Could you check a few things on this drawing? It's one solid part, dimensions in mm from its lowest x, y, z. Give positions to 0.01 mm unless a question says otherwise; leave off trailing zeros. Order: outer loops, then holes, each group sorted by start corner. A loop starts at its lowest first (then second) coordinate and runs counter-clockwise, first axis right, second up. Notation, with made-up numbers: (15.25, -37) -> (70.25, -37) arc R31 ccw to (70.25, -6) -> close; hole circle Ø10 at (61, 6). An arc over 180 degrees is marked (long way). Write each question's results on one line, items separated by ' | '. Start each with the question number.
Q1. I'm going to push flat-ended pins straight in: pin 1 (2 mm diameter, centred on x = 16, y = 23, fed in from +Z); pin 2 (1.5 mm diameter, centred on x = 64.5, y = 63.5, fed in from +Z). Where does each tip first touch, or does it pass through?
Q2. Imagine slicing it at C-C, the plane z = 0.8. Please give me the cut outline in (x, y).
Q3. Thinking about a two-plate mould opening in X: for the marked faces 1 and 2, which applies, pulls with the +X half, pulls with the -X half, needs draft (parallel to the pull), parting line crosses it, or undercut?
Q4. I need wall thicknesses on line 1 along X through (y, z) = (39, 0.65); line 2 along Y through (x, z) = (40, 0.95); line 3 along X through (y, z) = (15.5, 3.7). Which ranges of each line are inside material? Lowest first, please. Write a range as [from, to].
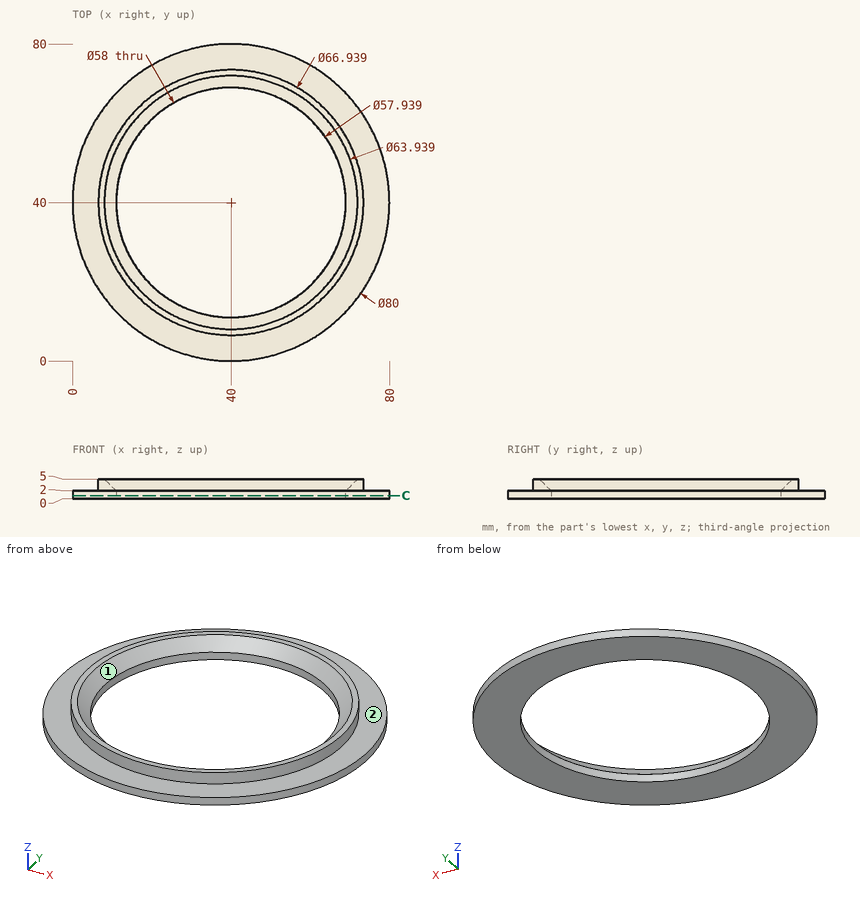
Geometry check:
1) pin 1: z = 3.44 | pin 2: z = 5
2) outline: circle Ø80 at (40, 40); hole circle Ø58 at (40, 40)
3) face 1: undercut | face 2: needs draft
4) line 1: [0.01, 11.02], [68.98, 79.99] | line 2: [0, 11], [69, 80] | line 3: [17.2, 21.55], [58.45, 62.8]
